Design review of the part shown in the three views and the two pictorial views. Dimensions are in mm from the part's minimum x, y and z. Give positions to 0.01 mm unless a question says otherwise; leave off trailing zeros. Write each loop counter-clockwise with the first axis right and the second up, starting at its lowest first coordinate (ties: lowest second). Pieces come first, ordered by that corner, then holes.
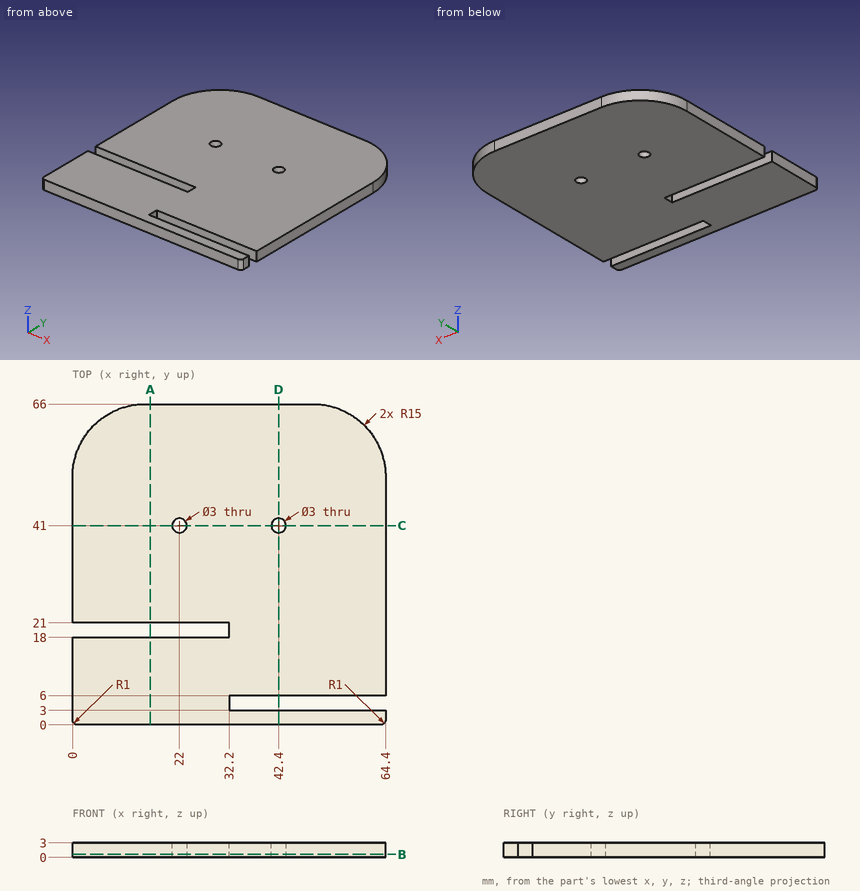
(1) Consider section C-C, the plane y = 41. Give the boundary of the cut face in (x, z).
Resolved:
outline: (0, 0) - (20.5, 0) - (20.5, 3) - (0, 3) - close; (23.5, 0) - (40.9, 0) - (40.9, 3) - (23.5, 3) - close; (43.9, 0) - (64.4, 0) - (64.4, 3) - (43.9, 3) - close
(2) Consider section A-A, the plane x = 16. Give the boundary of the cut face in (y, z), then the cut area to 3 significant figures.
Resolved:
outline: (0, 0) - (18, 0) - (18, 3) - (0, 3) - close; (21, 0) - (66, 0) - (66, 3) - (21, 3) - close
area: 189 mm2
(3) Consider section D-D, the plane x = 42.4. Give the boundary of the cut face in (y, z), then the cut area to 3 significant figures.
Resolved:
outline: (0, 0) - (3, 0) - (3, 3) - (0, 3) - close; (6, 0) - (39.5, 0) - (39.5, 3) - (6, 3) - close; (42.5, 0) - (66, 0) - (66, 3) - (42.5, 3) - close
area: 180 mm2
(4) Consider section B-B, the plane z = 0.65. Give the boundary of the cut face in (x, y).
Resolved:
outline: (0, 1) arc R1 ccw to (1, 0) - (63.4, 0) arc R1 ccw to (64.4, 1) - (64.4, 3) - (32.2, 3) - (32.2, 6) - (64.4, 6) - (64.4, 51) arc R15 ccw to (49.4, 66) - (15, 66) arc R15 ccw to (0, 51) - (0, 21) - (32.2, 21) - (32.2, 18) - (0, 18) - close; hole circle Ø3 at (22, 41); hole circle Ø3 at (42.4, 41)
(5) To check wall thickness, follow L1, parallel to Y at x = 42.4, z = 1.95; L2, parallel to Y at x = 22, z = 1.9; L3, parallel to X at y = 41, z = 1.9. State the ranges of each line that lie inside material, in increasing order.
Resolved:
L1: y = 0 to 3, 6 to 39.5, 42.5 to 66
L2: y = 0 to 18, 21 to 39.5, 42.5 to 66
L3: x = 0 to 20.5, 23.5 to 40.9, 43.9 to 64.4
(6) Clearance check with flat-ended pins moving along their axes: P1, Ø1.5, axis at x = 21.5, z = 1, coming from the -Y side; P2, Ø1.5, axis at y = 4.5, z = 1.5, coming from the +X side; P3, Ø1.5, axis at x = 55, z = 1, coming from the +Y side. State where each tip first meets the part, or that it passes through.
Resolved:
P1: stops at y = 0
P2: stops at x = 32.2
P3: stops at y = 65.19
